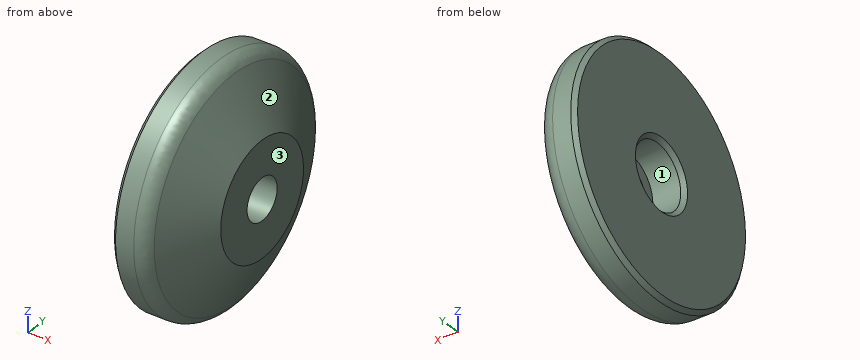
```python
from build123d import *

# Parameters (mm, degrees)
F2_R    = 2
F3_SIZE = 0.5


with BuildPart() as f1:
    # F0 (on Front) → F1 (revolve)
    with BuildSketch(Plane.XZ):
        Polygon((4, 15), (0, 15), (0, 4), (4, 4), (4, 2.6), (8, 2.6), (8, 7.149558), align=None)
    revolve(axis=Axis((12.800059, 0, 0), (1, 0, 0)))

    # F2
    f2_edges = [f1.edges().sort_by_distance(p)[0] for p in [
        (4, 0, -15),
    ]]
    fillet(f2_edges, radius=F2_R)

    # F3
    f3_edges = [f1.edges().sort_by_distance(p)[0] for p in [
        (0, 0, -4),
        (0, 0, -15),
    ]]
    chamfer(f3_edges, length=F3_SIZE)


solid = f1.part
```
For this review, take the finished solid that the model builds, in its own axes (mm). Face numbers are marked on the shaded views. Round coordinates to 2 decimals unless told otherwise and drop trailing zeros. Order: outer loops, then holes, each group sorted by start corner. A loop starts at its lowest first (then second) coordinate and runs counter-clockwise, first axis right, second up. Notation, with made-up numbers: (-25, -5.75) -> (-17, -5.75) arc R25 ccw to (-17, 23.25) -> close; hole circle Ø11 at (41.25, -38). An arc over 180 degrees is marked (long way). Use a Markdown table: item, result.
Item 1: Take a section at A-A (x = 5.75). State the section outline as (y, z) points.
Resolved:
| item | result |
|---|---|
| outline | circle Ø23.13 at (0, 0); hole circle Ø5.2 at (0, 0) |
Item 2: For pin 1 (5 mm diameter, centred on y = 0, z = 0, fed in from -X); pin 2 (6 mm diameter, centred on y = 0, z = 0, fed in from -X); pin 3 (1 mm diameter, centred on x = 2.5, z = -2, fed in from -Y), all flat-tipped, find the tip position at first contact; note any pin that passes through.
Resolved:
| item | result |
|---|---|
| pin 1 | passes through |
| pin 2 | stops at x = 4 |
| pin 3 | stops at y = -14.92 |
Item 3: For line 1 along Z through (x, y) = (1.4, 0); line 2 along Y through (x, z) = (6.65, 0); line 3 along X through (y, z) = (2, 2.5), list the stretches that pass through material, from the lowest coordinate up. Write a range as [from, to].
Resolved:
| item | result |
|---|---|
| line 1 | z = [-15, -4], [4, 15] |
| line 2 | y = [-9.8, -2.6], [2.6, 9.8] |
| line 3 | x = [4, 8] |
Item 4: Draft analysis for pull direction Z (two halves, no side actions). For the marked faces 1, 2 and 3, state which applies: +Z half, -Z half, draft (parallel to the pull), parting line (faces both ways), or undercut.
Resolved:
| item | result |
|---|---|
| face 1 | undercut |
| face 2 | parting line |
| face 3 | draft |
